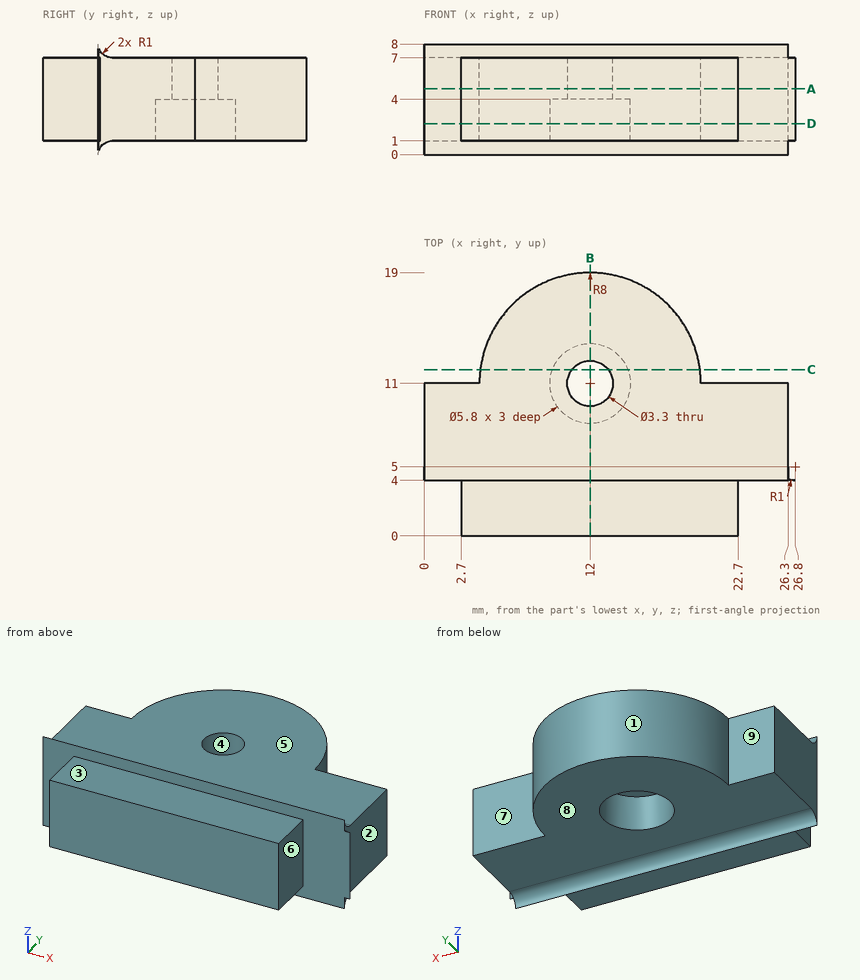
Answer from the drawing. Dimensions are ordinates in mm from the lowest x, y and z of the part. A direction names the side the tool comes from. Round coordinates to 2 decimals unless told otherwise and drop trailing zeros. Write each loop counter-clockwise with the first axis right and the second up, starting at its lowest first coordinate (ties: lowest second). Pieces come first, ordered by that corner, then holes. Notation, with made-up numbers: M -18,86 L -13,86 A21 ccw -13,122 Z; hole C 13.25,30.5 d9. An arc over 180 degrees is marked long. One line per item, written item: value.
Q1. Which of the six approach directions +Z, -Z, +X, -X, +Y, -Y give full straight-line access (tool end or side, diameter ignored) to the marked faces 5, 6, 7, 8 and 9?
Data:
face 5: +Z, +X, -X, +Y
face 6: +Z, -Z, +X, -Y
face 7: +Z, -Z, +X, +Y
face 8: -Z, +X, -X, +Y
face 9: +Z, -Z, -X, +Y
Q2. Find section D-D on z = 2.25. Write down the section's boundary in (x, y).
Data:
outline: M 0,4 L 2.7,4 L 2.7,0 L 22.7,0 L 22.7,4 L 26.8,4 A1 cw 26.3,4.13 L 26.3,11 L 20,11 A8 ccw 4,11 L 0,11 Z; hole C 12,11 d5.8
Q3. Flat-ended cylindrical pins translate along their axes: pin 1 Ø1.2 at (y, z) = (1.5, 2.5) entering from +X; pin 2 Ø2 at (y, z) = (14.5, 6) entering from -X; pin 3 Ø1 at (y, z) = (13.5, 1.5) entering from +X; pin 4 Ø2 at (x, z) = (3, 2) entering from -Y. Find the tip coordinate at first contact, or state that the pin passes through.
Data:
pin 1: x = 22.7
pin 2: x = 4.4
pin 3: x = 19.75
pin 4: y = 0
Q4. For a pull along X with two mould halves and no side action, classify the marked faces 1, 2, 3 and 4 as +X half, -X half, draft (parallel to the pull), parting line (faces both ways), or undercut.
Data:
face 1: parting line
face 2: +X half
face 3: draft
face 4: undercut
Q5. Find section B-B on x = 12. Write down the section's boundary in (y, z), plus the area to 3 significant figures.
Data:
outline: M 0,1 L 4,1 L 4,0 A1 cw 5,1 L 8.1,1 L 8.1,4 L 9.35,4 L 9.35,7 L 5,7 A1 cw 4,8 L 4,7 L 0,7 Z; M 12.65,4 L 13.9,4 L 13.9,1 L 19,1 L 19,7 L 12.65,7 Z
area: 87.1 mm2
Q6. Find section C-C on y = 12. Write down the section's boundary in (x, z).
Data:
outline: M 4.06,1 L 9.28,1 L 9.28,4 L 10.69,4 L 10.69,7 L 4.06,7 Z; M 13.31,4 L 14.72,4 L 14.72,1 L 19.94,1 L 19.94,7 L 13.31,7 Z
Q7. Straight lines are drawn through the part: line 1 (Y direction, x = 12, z = 4.8); line 2 (Y direction, x = 12, z = 2.9); line 3 (Z direction, x = 22.25, y = 6.5). For each, find the intervals that lie inside material, in ascending order. Write a range as [from, to].
Data:
line 1: [0, 9.35], [12.65, 19]
line 2: [0, 8.1], [13.9, 19]
line 3: [1, 7]
Q8. Find section A-A on z = 4.75. Write down the section's boundary in (x, y).
Data:
outline: M 0,4 L 2.7,4 L 2.7,0 L 22.7,0 L 22.7,4 L 26.8,4 A1 cw 26.3,4.13 L 26.3,11 L 20,11 A8 ccw 4,11 L 0,11 Z; hole C 12,11 d3.3
